Part model, mm, in its own coordinate system. A direction names the side the tool comes from. Round coordinates to 2 decimals unless told otherwise and drop trailing zeros. Order: outer loops, then holes, each group sorted by start corner. A loop starts at its lowest first (then second) coordinate and runs counter-clockwise, first axis right, second up. Notation, with made-up numbers: (19.25, 11) -> (70.25, 11) arc R19 cw to (70.25, 17) -> close; hole circle Ø7 at (5, 54). An arc over 180 degrees is marked (long way). Answer as a JSON object with one key per item and string values. Group by question number.
Autodesk Inventor part; units mm, degrees
ref_plane "YZ Plane" through (0, 0, 0) normal (1, 0, 0) x (0, 1, 0)
ref_plane "XZ Plane" through (0, 0, 0) normal (0, 1, 0) x (-1, 0, 0)
ref_plane "XY Plane" through (0, 0, 0) normal (0, 0, 1) x (1, 0, 0)
sketch "Sketch_1" plane through (0, 0, 0) normal (0, 0, 1) x (1, 0, 0)
  line L0 (6, 0) -> (-8.8, 0)
  line L1 (-8.8, 0) -> (-8.8, 5)
  line L2 (-8.8, 5) -> (-6, 5)
  line L3 (-6, 5) -> (-6, 3)
  line L4 (-6, 3) -> (0, 3)
  line L5 (0, 3) -> (0, 2)
  line L6 (0, 2) -> (5.5705, 2)
  line L7 (5.5705, 2) -> (6, 1.5705)
  line L8 (6, 1.5705) -> (6, 0)
  line L9 (6, 0) -> (-8.8, 0)
revolve "Revolution1" add sketch "Sketch_1" angle 360 about axis through (6, 0, 0) along (1, 0, 0)
thread "Thread1"
sketch "Sketch_2" plane through (-8.8, 0, 0) normal (-1, 0, 0) x (0, 1, 0)
  line L0 (-1.4434, 0) -> (-0.7217, -1.25)
  line L1 (-0.7217, -1.25) -> (0.7217, -1.25)
  line L2 (0.7217, -1.25) -> (1.4434, 0)
  line L3 (1.4434, 0) -> (0.7217, 1.25)
  line L4 (0.7217, 1.25) -> (-0.7217, 1.25)
  line L5 (-0.7217, 1.25) -> (-1.4434, 0)
extrude "Extrusion1" cut sketch "Sketch_2" against normal blind 2.5
sketch "Sketch_3" plane through (0, 0, 0) normal (0, 0, 1) x (1, 0, 0)
  line L0 (-5.5783, 0) -> (-6.3, 0)
  line L1 (-6.3, 0) -> (-6.3, 1.25)
  line L2 (-6.3, 1.25) -> (-5.5783, 0)
  line L3 (-5.5783, 0) -> (-6.3, 0)
revolve "Revolution2" cut sketch "Sketch_3" angle 360 about axis through (-5.5783, 0, 0) along (1, 0, 0)
properties part number "DBB4-6-6" material "스테인리스스틸"
Q1. Band-saw the part on A-A (x = -7.5). List the corners of the cut face in (y, z), plus the area to 3 significant figures.
Q2. Band-saw the part on C-C (y = 2.5). List the corners of the cut face in (x, z).
Q3. Wall check: line 1 (X direction, y = 1, z = 3); line 2 (X direction, y = 0.75, z = 2); line 3 (Z direction, x = -2, y = 0). Give the ranges that are in metal, low to high. Write a range as [from, to].
Q4. Which spindle directions (+Z, -Z, +X, -X, +Y, -Y) get a long thin tool onto all of the face, cutting with end or side? Do faces 5 (the flat face through (-8, 0, 1.25)), 6 (the flat face through (6, 0, 0)), 7 (the flat face through (0, 1, -2)). Say none if no direction does.
Q5. Band-saw the part on D-D (x = -4.25). List the corners of the cut face in (y, z).
Q6. Drop flat-ended pins along their axis: pin 1 Ø1.5 at (x, z) = (-5, -1.5) entering from +Y; pin 2 Ø6 at (x, z) = (-1.5, 2.5) entering from +Y; pin 3 Ø1.5 at (y, z) = (-2.5, -3.5) entering from +X. Give the stop position or say it passes through.
Q7. Two-plate mould, pull along Z, no slides. Class faces 1 (the flat face through (-8.8, 1.04, -1.04)), 2 (the cylindrical face through (-3, -3, 0)), 3 (the flat face through (-8, 0, -1.25)), 4 (the flat face through (-7.57, -1.08, -0.63)): +Z half, -Z half, draft (parallel to the pull), parting line (faces both ways), or undercut.
Q8. Band-saw the part on B-B (z = 2.75). List the corners of the cut face in (x, y), plus the area to 3 significant figures.
Completed:
{
 "1": {"outline": "circle Ø10 at (0, 0); hole (-1.44, 0) -> (-0.72, -1.25) -> (0.72, -1.25) -> (1.44, 0) -> (0.72, 1.25) -> (-0.72, 1.25) -> close", "area": "73.1 mm2"},
 "2": {"outline": "(-8.8, -4.33) -> (-6, -4.33) -> (-6, -1.66) -> (0, -1.66) -> (0, 1.66) -> (-6, 1.66) -> (-6, 4.33) -> (-8.8, 4.33) -> close"},
 "3": {"line 1": "[-8.8, -6]", "line 2": "[-8.8, 0]", "line 3": "[-3, 3]"},
 "4": {"face 5": "-X", "face 6": "+Z, -Z, +X, +Y, -Y", "face 7": "+X"},
 "5": {"outline": "circle Ø6 at (0, 0)"},
 "6": {"pin 1": "y = 2.9", "pin 2": "y = 3", "pin 3": "x = -6"},
 "7": {"face 1": "draft", "face 2": "parting line", "face 3": "undercut", "face 4": "undercut"},
 "8": {"outline": "(-8.8, -4.18) -> (-6, -4.18) -> (-6, -1.2) -> (0, -1.2) -> (0, 1.2) -> (-6, 1.2) -> (-6, 4.18) -> (-8.8, 4.18) -> close", "area": "37.8 mm2"}
}
